```python
from build123d import *

# Parameters (mm, degrees)
F0_R     = 127
F1_DEPTH = 3.175
F2_R     = 0.508
F3_R     = 123.19
F4_DEPTH = 1.27


with BuildPart() as f1:
    # F0 (on Top) → F1 (new body)
    with BuildSketch(Plane.XY):
        Circle(F0_R)
    extrude(amount=F1_DEPTH)

    # F2
    f2_edges = [f1.edges().sort_by_distance(p)[0] for p in [
        (-127, 0, 0),
        (-127, 0, 3.175),
    ]]
    fillet(f2_edges, radius=F2_R)

    # F3 (on face) → F4 (cut)
    with BuildSketch(Plane.XY.offset(3.175)):
        Circle(F3_R)
    extrude(amount=-F4_DEPTH, mode=Mode.SUBTRACT)


solid = f1.part
```
Geometry: final body of the model. Coordinates: model frame, mm. A direction names the side the tool comes from. Coordinates: 2 decimals unless noted, no trailing zeros. Write each loop counter-clockwise with the first axis right and the second up, starting at its lowest first coordinate (ties: lowest second). Pieces come first, ordered by that corner, then holes. Notation, with made-up numbers: M -2.5,-11 L 54.5,-11 A25 ccw 54.5,16 Z; hole C 70.25,60.25 d6. An arc over 180 degrees is marked long. Use CSV: the item, a comma, the result in double quotes. Start each with the question number.
1. Cut plane A-A on x = 0. Return the cut outline in (y, z) (3 decimals).
2. Ray query, probe 1 along Y at (x, z) = (0, 2.75); probe 2 along Z at (x, y) = (-38.5, -47) (3 decimals); probe 3 along Y at (x, z) = (-71.5, 2.1). Return the intervals inside material, ascending.
3. Mould query, pull axis X, two halves, no side actions, for faces 1 (the face through (28, -121, 3.175)), 2 (the face through (-27.53, -123.98, 1.57)), 3 (the face through (-26.71, -120.26, 2.55)). Classes: pulls with the +X half, pulls with the -X half, needs draft (parallel to the pull), parting line crosses it, or undercut.
4. Reachability of faces 4 (the face through (-2, 2, 1.905)), 5 (the face through (-2, 2, 0)) from +Z, -Z, +X, -X, +Y, -Y: full face, straight path, thin tool, end or side. Return the list, or none.
5. First-contact query: P1, Ø1.5, axis at x = 10.5, z = 1.5, coming from the +Y side; P2, Ø1, axis at y = -9.5, z = 2, coming from the +X side; P3, Ø10, axis at x = 13.5, y = -38, coming from the +Z side (3 decimals); P4, Ø1.5, axis at x = 91, y = 90.5, coming from the -Z side. Flat tips, straight axial feed; report the tip coordinate or a pass-through.
Entries:
1,outline,"M -127,0.508 A0.508 ccw -126.492,0 L 126.492,0 A0.508 ccw 127,0.508 L 127,2.667 A0.508 ccw 126.492,3.175 L 123.19,3.175 L 123.19,1.905 L -123.19,1.905 L -123.19,3.175 L -126.492,3.175 A0.508 ccw -127,2.667 Z"
2,probe 1,"-126.99 to -123.19, 123.19 to 126.99"
2,probe 2,"0 to 1.905"
2,probe 3,"-104.96 to -100.32, 100.32 to 104.96"
3,face 1,"needs draft"
3,face 2,"parting line crosses it"
3,face 3,"undercut"
4,face 4,"+Z"
4,face 5,"-Z, +X, -X, +Y, -Y"
5,P1,"y = 126.63"
5,P2,"x = 126.68"
5,P3,"z = 1.905"
5,P4,"through"
